Geometry check sheet. Reference: the model listing, model coordinates, mm. A direction names the side the tool comes from. Round coordinates to 2 decimals unless told otherwise and drop trailing zeros. Order: outer loops, then holes, each group sorted by start corner. A loop starts at its lowest first (then second) coordinate and runs counter-clockwise, first axis right, second up. Notation, with made-up numbers: (16.25, 31.25) -> (50.25, 31.25) arc R11 cw to (50.25, 35.25) -> close; hole circle Ø3 at (12.25, -14.5). An arc over 180 degrees is marked (long way). Answer as a JSON object with one key per item and string values. Group by question number.
Autodesk Fusion 360 part; units mm, degrees
sketch "草图1" plane through (0, 0, 0) normal (0, 1, 0) x (1, 0, 0)
  line L0 (0, 0) -> (5, 0)
  line L1 (5, 0) -> (5, 9.6)
  line L2 (5, 9.6) -> (0, 9.6)
  line L3 (0, 9.6) -> (0, 0)
  circle A0 centre (2.5, 2.5) radius 2.5
  circle A1 centre (2.5, 7.1) radius 2.5
  dimension "d1" = 5
  dimension "d2" = 9.6
  dimension "d3" = 5
  dimension "d4" = 5
extrude "拉伸1" add sketch "草图1" along normal blind 1 contours A0 A1 | L3 A0 A1 | L1 A0 A1 | A0 A1 | A0 A1
sketch "草图2" plane through (0, 1, 0) normal (0, 1, 0) x (-1, 0, 0)
  line L0 (1.0001, 5.2) -> (-5.9999, 5.2)
  line L1 (-5.9999, 5.2) -> (-5.9999, -14.8)
  line L2 (-5.9999, -14.8) -> (1.0001, -14.8)
  line L3 (1.0001, -14.8) -> (1.0001, 5.2)
  line L4 (8, -4.8) -> (-8, -4.8)
  line L5 (0, -7.1) -> (0, -2.5)
  line L6 (-2.4999, 15.7777) -> (-2.4999, -15.7777)
  arc A0 (0, -2.5) -> (-5, -2.4998) centre (-2.5, -2.5) ccw
  line L7 (-5.9999, 5.2) -> (1.0001, -14.8)
  line L8 (1.0001, 5.2) -> (-5.9999, -14.8)
  circle A1 centre (-2.4999, -4.8) radius 1.267
  circle A2 centre (-2.4999, -4.8) radius 1.114
  circle A3 centre (-2.4999, 1.7) radius 3.5
  circle A4 centre (-2.4999, -11.3) radius 3.5
  line L9 (1.0001, 5.2) -> (1.0001, 0)
  line L10 (1.0001, 0) -> (1.4001, 0)
  line L11 (1.4001, 0) -> (1.4001, -9.6)
  line L12 (1.4001, -9.6) -> (1.0001, -9.6)
  dimension "d11" = 7
  dimension "d12" = 20
  dimension "d13" = 7
  dimension "d14" = 7
  dimension "d15" = 5.2
  dimension "d19" = 0.4
  dimension "d20" = 9.6
extrude "拉伸2" add sketch "草图2" along normal blind 2.65 contours L6 A0 L8 A3 | L6 A0 L7 A3 | A0 L8 A3 | L3 L4 L5 A0 A3 L9 | L6 A0 L8 A3 | L6 A0 L7 A3 | A0 L7 A3 | A0 L8 A3 | L4 L5 A0 L8 A1 A3 | L1 L4 L7 A1 A3 | L6 L8 A1 A3 | L6 L7 A1 A3 | A0 L7 A3 | L3 L4 L7 A1 A4 | L1 L4 L8 A1 A4 | L6 L8 A1 A2 | L6 L7 A1 A2 | L4 L8 A1 A2 | L8 A4 | L4 L7 A1 A2 | L4 L8 A1 A2 | L6 L8 A2 | L6 L7 A2 | L7 A4 | L4 L7 A1 A2 | L4 L8 A2 | L6 L8 A4 | L6 L8 A1 A4 | L4 L7 A2 | L4 L8 A2 | L6 L8 A1 A2 | L6 L7 A2 | L4 L7 A2 | L6 L8 A2 | L6 L7 A1 A4 | L6 L7 A4 | L6 L7 A1 A2
sketch "草图3" plane through (0, 3.65, 0) normal (0, 1, 0) x (-1, 0, 0)
  arc A0 (1.0001, 1.7) -> (-5.9999, 1.7) centre (-2.4999, 1.7) ccw
  line L0 (-5.9999, 1.7) -> (-5.9999, -11.3)
  arc A1 (-5.9999, -11.3) -> (1.0001, -11.3) centre (-2.4999, -11.3) ccw
  line L1 (1.0001, -11.3) -> (1.0001, 1.7)
  line L2 (3.0001, -4.8) -> (-14.9999, -4.8)
  line L3 (-5.9999, 2.4) -> (-5.9999, -12)
  line L4 (-2.4999, 10.5811) -> (-2.4999, -40.1811)
  line L5 (-5.9999, 2.4) -> (-2.4999, 2.4)
  line L6 (-5.9999, -12) -> (-2.4999, -12)
  circle A2 centre (-2.4999, 2.4) radius 1
  circle A3 centre (-2.4999, -12) radius 1
  dimension "d24" = 14.4
  dimension "d25" = 2
  dimension "d26" = 2
extrude "拉伸3" cut sketch "草图3" against normal blind 2.65 contours L4 A2 | L4 L5 A2 | L4 L5 A2 | L4 A3 | L4 L6 A3 | L4 L6 A3
sketch "草图5" plane through (0, 3.65, 0) normal (0, 1, 0) x (-1, 0, 0)
  circle A0 centre (-2.4999, 2.4) radius 1
  circle A1 centre (-2.4999, -12) radius 1
  arc A2 (1.0001, 1.7) -> (-5.9999, 1.7) centre (-2.4999, 1.7) ccw
  line L0 (-5.9999, 1.7) -> (-5.9999, -11.3)
  arc A3 (-5.9999, -11.3) -> (1.0001, -11.3) centre (-2.4999, -11.3) ccw
  line L1 (1.0001, -11.3) -> (1.0001, 1.7)
  line L2 (2.5, 5.2) -> (-8.5, 5.2)
  line L3 (1.0001, 1.7) -> (1.0001, 5.2)
  line L4 (-5.9999, 1.7) -> (-5.9999, 5.2)
  line L5 (1.0001, 5.2) -> (1.0001, 0)
  line L6 (-5.9999, 5.2) -> (-5.9999, 0.2)
  line L7 (1.0001, 0) -> (1.4001, 0)
  line L8 (1.4001, 0) -> (1.4001, -9.6)
  line L9 (1.4001, -9.6) -> (1.0001, -9.6)
  line L10 (1.0001, -9.6) -> (1.0001, 0)
  line L11 (-5.9999, 0.2) -> (-11.9999, 0.2)
  line L12 (-11.9999, 0.2) -> (-11.9999, -9.8)
  line L13 (-11.9999, -9.8) -> (-5.9999, -9.8)
  line L14 (-5.9999, -9.8) -> (-5.9999, 0.2)
  dimension "d37" = 5.2
  dimension "d38" = 5
  dimension "d39" = 0.4
  dimension "d40" = 9.6
  dimension "d41" = 6
  dimension "d42" = 10
extrude "拉伸4" add sketch "草图5" against normal blind 1 contours L1 L7 L8 L9 L10 | L0 L11 L12 L13 L14
sketch "草图6" plane through (0, 3.65, 0) normal (0, 1, 0) x (-1, 0, 0)
  circle A0 centre (-2.4999, 2.4) radius 1
  circle A1 centre (-2.4999, -12) radius 1
  arc A2 (1.0001, 1.7) -> (-5.9999, 1.7) centre (-2.4999, 1.7) ccw
  line L0 (-5.9999, 1.7) -> (-5.9999, 0.2)
  line L1 (-5.9999, 0.2) -> (-11.9999, 0.2)
  line L2 (-11.9999, 0.2) -> (-11.9999, -9.8)
  line L3 (-11.9999, -9.8) -> (-5.9999, -9.8)
  line L4 (-5.9999, -9.8) -> (-5.9999, -11.3)
  arc A3 (-5.9999, -11.3) -> (1.0001, -11.3) centre (-2.4999, -11.3) ccw
  line L5 (1.0001, -11.3) -> (1.0001, -9.6)
  line L6 (1.0001, -9.6) -> (1.4001, -9.6)
  line L7 (1.4001, -9.6) -> (1.4001, 0)
  line L8 (1.4001, 0) -> (1.0001, 0)
  line L9 (1.0001, 0) -> (1.0001, 1.7)
  line L10 (-11.9999, 0.2) -> (-10.9999, 0.2)
  line L11 (-10.9999, 0.2) -> (-10.9999, -0.8)
  line L12 (-10.9999, -0.8) -> (-11.9999, -0.8)
  line L13 (-11.9999, -0.8) -> (-11.9999, 0.2)
  line L14 (-10.9999, -0.8) -> (-7.1624, -0.8)
  line L15 (-7.1624, -0.8) -> (-7.1624, -8.8)
  line L16 (-7.1624, -8.8) -> (-10.9999, -8.8)
  line L17 (-10.9999, -8.8) -> (-10.9999, -0.8)
  dimension "d46" = 1
  dimension "d47" = 1
  dimension "d48" = 8
extrude "拉伸5" add sketch "草图6" along normal blind 3 contours L14 L15 L16 L17
sketch "草图7" plane through (10.9999, 0, 0) normal (1, 0, 0) x (0, 0, -1)
  line L0 (0.8, 3.65) -> (8.8, 3.65)
  line L1 (8.8, 3.65) -> (8.8, 6.65)
  line L2 (8.8, 6.65) -> (0.8, 6.65)
  line L3 (0.8, 6.65) -> (0.8, 3.65)
  line L4 (0.8, 6.65) -> (1.2, 6.65)
  line L5 (1.2, 6.65) -> (1.2, 6.25)
  line L6 (1.2, 6.25) -> (0.8, 6.25)
  line L7 (0.8, 6.25) -> (0.8, 6.65)
  line L8 (8.8, 3.65) -> (8.4, 3.65)
  line L9 (8.4, 3.65) -> (8.4, 4.05)
  line L10 (8.4, 4.05) -> (8.8, 4.05)
  line L11 (8.8, 4.05) -> (8.8, 3.65)
  line L12 (1.2, 6.25) -> (8.4, 6.25)
  line L13 (8.4, 6.25) -> (8.4, 4.05)
  line L14 (8.4, 4.05) -> (1.2, 4.05)
  line L15 (1.2, 4.05) -> (1.2, 6.25)
  line L16 (1.2, 6.0193) -> (8.4, 6.0193)
  line L17 (1.2, 5.7535) -> (8.4, 5.7535)
  line L18 (1.2, 5.7535) -> (1.05, 5.7535)
  line L19 (1.2, 6.0193) -> (1.05, 6.0193)
  line L20 (1.05, 6.0193) -> (1.05, 5.7535)
  line L21 (4.8, 10.0193) -> (4.8, 2.0193)
  line L22 (8.55, 5.7535) -> (8.4, 5.7535)
  line L23 (8.55, 6.0193) -> (8.4, 6.0193)
  line L24 (8.55, 5.7535) -> (8.55, 6.0193)
  point P0 (8.55, 6.0193)
  point P1 (8.55, 5.7535)
  dimension "d51" = 0.4
  dimension "d52" = 0.4
  dimension "d53" = 0.4
  dimension "d54" = 0.4
  dimension "d55" = 0.15
  dimension "d56" = 0.15
extrude "拉伸6" cut sketch "草图7" against normal blind 3.438 contours L13 L14 L17 L21 | L14 L15 L17 L21 | L13 L16 L17 L21 | L13 L22 L23 L24 | L15 L16 L17 L21 | L12 L13 L16 L21 | L12 L15 L16 L21 | L15 L18 L19 L20
Item 1: Sectioned sample at A-A, the plane x = 8.5. Enter the section's corners in (y, z).
Item 2: Sectioned sample at B-B, the plane z = -5.5. Enter the section's corners in (x, y).
Item 3: Set-up check for faces 1 (the cylindrical face through (2.4, 0.5, -9.6)), 2 (the flat face through (0, 0.5, -4.8)), 3 (the flat face through (9, 5, -0.8)): record each of +Z, -Z, +X, -X, +Y, -Y from which the full face is reachable in a straight line by a thin tool's end or side.
Item 4: Depth check by flat-ended pin: pin 1 Ø1.1 at (y, z) = (5, -6.5) entering from +X; pin 2 Ø1.5 at (x, y) = (1.5, 1.5) entering from +Z; pin 3 Ø1.7 at (x, z) = (9.5, -4) entering from -Y; pin 4 Ø3 at (y, z) = (5.5, -11) entering from +X. Enter the tip coordinate at first touch or a pass-through.
Item 5: Sectioned sample at D-D, the plane x = 3. Enter the section's corners in (y, z).
Item 6: Sectioned sample at C-C, the plane y = 2.25. Enter the section's corners in (x, z).
Item 7: Thickness scan on L1, parallel to Y at x = 10.5, z = -5.25; L2, parallel to Y at x = 7.5, z = -1; L3, parallel to Y at x = 6.75, z = -2.5. Record the ranges inside material, lowest first.
Item 8: Mould release check, pull along Y, two halves, no side actions. Record for faces 4 (the flat face through (9, 4.05, -5)), 5 (the flat face through (2, 0, -5)), 6 (the flat face through (9, 3, 0.2)), 7 (the flat face through (9, 5, -1.2)): pulls with the +Y half, pulls with the -Y half, needs draft (parallel to the pull), parting line crosses it, or undercut.
Result:
{
 "1": {"outline": "(2.65, -9.8) -> (3.65, -9.8) -> (3.65, -8.8) -> (6.65, -8.8) -> (6.65, -0.8) -> (3.65, -0.8) -> (3.65, 0.2) -> (2.65, 0.2) -> close; hole (4.05, -8.4) -> (5.75, -8.4) -> (5.75, -8.55) -> (6.02, -8.55) -> (6.02, -8.4) -> (6.25, -8.4) -> (6.25, -1.2) -> (6.02, -1.2) -> (6.02, -1.05) -> (5.75, -1.05) -> (5.75, -1.2) -> (4.05, -1.2) -> close"},
 "2": {"outline": "(-1.4, 2.65) -> (-1, 2.65) -> (-1, 1) -> (0, 1) -> (0, 0) -> (5, 0) -> (5, 1) -> (6, 1) -> (6, 2.65) -> (12, 2.65) -> (12, 3.65) -> (11, 3.65) -> (11, 4.05) -> (7.56, 4.05) -> (7.56, 6.25) -> (11, 6.25) -> (11, 6.65) -> (7.16, 6.65) -> (7.16, 3.65) -> (-1.4, 3.65) -> close"},
 "3": {"face 1": "-Z, -Y", "face 2": "+Z, -Z, -X, -Y", "face 3": "+Z, +X, -X, +Y"},
 "4": {"pin 1": "stops at x = 7.56", "pin 2": "stops at z = 5.19", "pin 3": "stops at y = 2.65", "pin 4": "passes through"},
 "5": {"outline": "(0, -9.55) -> (1, -9.55) -> (1, -11.13) -> (3.65, -11.13) -> (3.65, 1.53) -> (1, 1.53) -> (1, -0.05) -> (0, -0.05) -> close; (1, -14.76) -> (3.65, -14.76) -> (3.65, -12.87) -> (1, -12.87) -> close; (1, 3.27) -> (3.65, 3.27) -> (3.65, 5.16) -> (1, 5.16) -> close"},
 "6": {"outline": "(-1, -11.3) arc R3.5 ccw to (6, -11.3) -> (6, 1.7) arc R3.5 ccw to (-1, 1.7) -> close; hole circle Ø2 at (2.5, -12); hole circle Ø2 at (2.5, 2.4)"},
 "7": {"L1": "y = 2.65 to 4.05, 6.25 to 6.65", "L2": "y = 2.65 to 6.65", "L3": "y = 2.65 to 3.65"},
 "8": {"face 4": "undercut", "face 5": "pulls with the -Y half", "face 6": "needs draft", "face 7": "undercut"}
}
